from build123d import *

# Parameters (mm, degrees)
SKETCH1_R                = 19.05
BOSS_EXTRUDE1_DEPTH      = 203.2
SKETCH2_R                = 33.02
BOSS_EXTRUDE2_DEPTH      = 1
BOSS_EXTRUDE3_START      = 1.016
SKETCH3_R                = 33.02
BOSS_EXTRUDE3_DEPTH      = 1.016
SHELL2_START             = -0.016
SHELL2_OUTLINE_R         = 18.05
SHELL2_DEPTH             = 204.216
BOSS_EXTRUDE4_REACH      = 235.917
BOSS_EXTRUDE4_END_RADIUS = 19.05
SKETCH4_R                = 6.35
CUT_EXTRUDE1_REACH       = 235.917
CUT_EXTRUDE1_END_RADIUS  = 18.05
SKETCH5_R                = 5.08
BOSS_EXTRUDE5_REACH      = 258.931
BOSS_EXTRUDE5_END_RADIUS = 19.05
SKETCH6_R                = 6.35
CUT_EXTRUDE3_REACH       = 223.383
SKETCH8_R                = 4
BOSS_EXTRUDE6_START      = 50.8
SKETCH9_R                = 6.35
BOSS_EXTRUDE6_DEPTH      = 255.016
CUT_EXTRUDE2_REACH       = 258.931
CUT_EXTRUDE2_END_RADIUS  = 18.05
SKETCH7_R                = 5.08
SKETCH11_R               = 44.45
BOSS_EXTRUDE7_DEPTH      = 1
CUT_EXTRUDE5_REACH       = 272.789
SKETCH13_R               = 2.032
CUT_EXTRUDE6_REACH       = 272.789
SKETCH15_R               = 5.08
FILLET1_R                = 0.254


# Read off the part's stored shape, not the designer's step: Shell2
with BuildPart() as part:
    # Sketch1 → Boss-Extrude1 (new body)
    with BuildSketch(Plane(origin=(0, 0, 0), x_dir=(1, 0, 0), z_dir=(0, 1, 0))):
        with Locations(Location((0, 0, 0), (0, 0, 270))):
            Circle(SKETCH1_R)
    extrude(amount=BOSS_EXTRUDE1_DEPTH)

    # Sketch2 → Boss-Extrude2 (add)
    with BuildSketch(Plane(origin=(0, 203.2, 0), x_dir=(1, 0, 0), z_dir=(0, 1, 0))):
        with Locations(Location((0, 0, 0), (0, 0, 270))):
            Circle(SKETCH2_R)
    extrude(amount=BOSS_EXTRUDE2_DEPTH)

    # Sketch3 → Boss-Extrude3 (add)
    with BuildSketch(Plane.XZ.offset(BOSS_EXTRUDE3_START)):
        with Locations(Location((0, 0, 0), (0, 0, 90))):
            Circle(SKETCH3_R)
    extrude(amount=-BOSS_EXTRUDE3_DEPTH)

    # Shell2 outline → Shell2 (cut)
    with BuildSketch(Plane(origin=(0, 0, 0), x_dir=(1, 0, 0), z_dir=(0, 1, 0)).offset(SHELL2_START)):
        Circle(SHELL2_OUTLINE_R)
    extrude(amount=SHELL2_DEPTH, mode=Mode.SUBTRACT)

    # Boss-Extrude4: up to this cylinder (the profile starts outside it)
    boss_extrude4_end = Plane(origin=(0, 189.341, 0), z_dir=(0, -1, 0)) * Cylinder(BOSS_EXTRUDE4_END_RADIUS, 510.934, mode=Mode.PRIVATE)
    # Sketch4 → Boss-Extrude4 (add, up to the surface)
    with BuildSketch(Plane(origin=(-76.2, 0, 0), x_dir=(0, 0, -1), z_dir=(1, 0, 0)), mode=Mode.PRIVATE) as boss_extrude4_sk1:
        with Locations(Location((0, 189.341, 0), (0, 0, 180))):
            Circle(SKETCH4_R)
    boss_extrude4_tool1 = extrude(boss_extrude4_sk1.sketch, amount=BOSS_EXTRUDE4_REACH, mode=Mode.PRIVATE) - boss_extrude4_end
    add(boss_extrude4_tool1.solids().sort_by_distance((-76.2, 189.341, 0))[0])

    # Cut-Extrude1: up to this cylinder (the profile starts outside it)
    cut_extrude1_end = Plane(origin=(0, 189.341, 0), z_dir=(0, -1, 0)) * Cylinder(CUT_EXTRUDE1_END_RADIUS, 508.934, mode=Mode.PRIVATE)
    # Sketch5 → Cut-Extrude1 (cut, up to the surface)
    with BuildSketch(Plane.ZY.offset(76.2), mode=Mode.PRIVATE) as cut_extrude1_sk1:
        with Locations((0, 189.341)):
            Circle(SKETCH5_R)
    cut_extrude1_tool1 = extrude(cut_extrude1_sk1.sketch, amount=-CUT_EXTRUDE1_REACH, mode=Mode.PRIVATE) - cut_extrude1_end
    add(cut_extrude1_tool1.solids().sort_by_distance((-76.2, 189.341, 0))[0], mode=Mode.SUBTRACT)

    # Boss-Extrude5: up to this cylinder (the profile starts outside it)
    boss_extrude5_end = Plane(origin=(0, 10.16, 0), z_dir=(0, -1, 0)) * Cylinder(BOSS_EXTRUDE5_END_RADIUS, 556.962, mode=Mode.PRIVATE)
    # Sketch6 → Boss-Extrude5 (add, up to the surface)
    with BuildSketch(Plane(origin=(76.2, 0, 0), x_dir=(0, 0, -1), z_dir=(1, 0, 0)), mode=Mode.PRIVATE) as boss_extrude5_sk1:
        with Locations((0, 10.16)):
            Circle(SKETCH6_R)
    boss_extrude5_tool1 = extrude(boss_extrude5_sk1.sketch, amount=-BOSS_EXTRUDE5_REACH, mode=Mode.PRIVATE) - boss_extrude5_end
    add(boss_extrude5_tool1.solids().sort_by_distance((76.2, 10.16, 0))[0])

    # Sketch8 → Cut-Extrude3 (cut, up to next)
    with BuildSketch(Plane.XZ.offset(1.016), mode=Mode.PRIVATE) as cut_extrude3_sk1:
        with Locations(Location((0, 0, 0), (0, 0, 270))):
            Circle(SKETCH8_R)
    cut_extrude3_tool1 = extrude(cut_extrude3_sk1.sketch, amount=-CUT_EXTRUDE3_REACH, mode=Mode.PRIVATE) & part.part
    add(cut_extrude3_tool1.solids().sort_by_distance((0, -1.016, 0))[0], mode=Mode.SUBTRACT)

    # Sketch9 → Boss-Extrude6 (add)
    with BuildSketch(Plane.XZ.offset(1.016).offset(BOSS_EXTRUDE6_START)):
        with Locations(Location((0, 0, 0), (0, 0, 270))):
            Circle(SKETCH9_R)
    extrude(amount=-BOSS_EXTRUDE6_DEPTH)

    # Cut-Extrude2: up to this cylinder (the profile starts outside it)
    cut_extrude2_end = Plane(origin=(0, 10.16, 0), z_dir=(0, -1, 0)) * Cylinder(CUT_EXTRUDE2_END_RADIUS, 554.962, mode=Mode.PRIVATE)
    # Sketch7 → Cut-Extrude2 (cut, up to the surface)
    with BuildSketch(Plane(origin=(76.2, 0, 0), x_dir=(0, 0, -1), z_dir=(1, 0, 0)), mode=Mode.PRIVATE) as cut_extrude2_sk1:
        with Locations((0, 10.16)):
            Circle(SKETCH7_R)
    cut_extrude2_tool1 = extrude(cut_extrude2_sk1.sketch, amount=-CUT_EXTRUDE2_REACH, mode=Mode.PRIVATE) - cut_extrude2_end
    add(cut_extrude2_tool1.solids().sort_by_distance((76.2, 10.16, 0))[0], mode=Mode.SUBTRACT)

    # Sketch11 → Boss-Extrude7 (add)
    with BuildSketch(Plane(origin=(0, 204.2, 0), x_dir=(1, 0, 0), z_dir=(0, 1, 0))):
        with Locations(Location((0, 0, 0), (0, 0, 270))):
            Circle(SKETCH11_R)
    extrude(amount=-BOSS_EXTRUDE7_DEPTH)

    # Sketch13 → Cut-Extrude5 (cut, up to next)
    with BuildSketch(Plane(origin=(0, 204.2, 0), x_dir=(1, 0, 0), z_dir=(0, 1, 0)), mode=Mode.PRIVATE) as cut_extrude5_sk1:
        with Locations(Location((33.02, 0, 0), (0, 0, 270))):
            Circle(SKETCH13_R)
    cut_extrude5_tool1 = extrude(cut_extrude5_sk1.sketch, amount=-CUT_EXTRUDE5_REACH, mode=Mode.PRIVATE) & part.part
    # Sketch13 → Cut-Extrude5 (cut, up to next)
    with BuildSketch(Plane(origin=(0, 204.2, 0), x_dir=(1, 0, 0), z_dir=(0, 1, 0)), mode=Mode.PRIVATE) as cut_extrude5_sk2:
        with Locations(Location((0, -33.02, 0), (0, 0, 270))):
            Circle(SKETCH13_R)
    cut_extrude5_tool2 = extrude(cut_extrude5_sk2.sketch, amount=-CUT_EXTRUDE5_REACH, mode=Mode.PRIVATE) & part.part
    # Sketch13 → Cut-Extrude5 (cut, up to next)
    with BuildSketch(Plane(origin=(0, 204.2, 0), x_dir=(1, 0, 0), z_dir=(0, 1, 0)), mode=Mode.PRIVATE) as cut_extrude5_sk3:
        with Locations(Location((-33.02, 0, 0), (0, 0, 270))):
            Circle(SKETCH13_R)
    cut_extrude5_tool3 = extrude(cut_extrude5_sk3.sketch, amount=-CUT_EXTRUDE5_REACH, mode=Mode.PRIVATE) & part.part
    # Sketch13 → Cut-Extrude5 (cut, up to next)
    with BuildSketch(Plane(origin=(0, 204.2, 0), x_dir=(1, 0, 0), z_dir=(0, 1, 0)), mode=Mode.PRIVATE) as cut_extrude5_sk4:
        with Locations(Location((0, 33.02, 0), (0, 0, 270))):
            Circle(SKETCH13_R)
    cut_extrude5_tool4 = extrude(cut_extrude5_sk4.sketch, amount=-CUT_EXTRUDE5_REACH, mode=Mode.PRIVATE) & part.part
    add(cut_extrude5_tool1.solids().sort_by_distance((33.02, 204.2, 0))[0], mode=Mode.SUBTRACT)
    add(cut_extrude5_tool2.solids().sort_by_distance((0, 204.2, 33.02))[0], mode=Mode.SUBTRACT)
    add(cut_extrude5_tool3.solids().sort_by_distance((-33.02, 204.2, 0))[0], mode=Mode.SUBTRACT)
    add(cut_extrude5_tool4.solids().sort_by_distance((0, 204.2, -33.02))[0], mode=Mode.SUBTRACT)

    # Sketch15 → Cut-Extrude6 (cut, up to next)
    with BuildSketch(Plane.XZ.offset(51.816), mode=Mode.PRIVATE) as cut_extrude6_sk1:
        with Locations(Location((0, 0, 0), (0, 0, 270))):
            Circle(SKETCH15_R)
    cut_extrude6_tool1 = extrude(cut_extrude6_sk1.sketch, amount=-CUT_EXTRUDE6_REACH, mode=Mode.PRIVATE) & part.part
    add(cut_extrude6_tool1.solids().sort_by_distance((0, -51.816, 0))[0], mode=Mode.SUBTRACT)

    # Fillet1
    fillet1_edges = [part.edges().sort_by_distance(p)[0] for p in [
        (0, 204.2, 5.08),
    ]]
    fillet(fillet1_edges, radius=FILLET1_R)


solid = part.part
Check sheet for the modelled part. Datum: model origin and axes. Units: mm. A direction names the side the tool comes from. Round coordinates to 2 decimals unless told otherwise and drop trailing zeros. Order: outer loops, then holes, each group sorted by start corner. A loop starts at its lowest first (then second) coordinate and runs counter-clockwise, first axis right, second up.
(1) Cross-section at B-B, the plane z = 22. Enter the section's corners in (x, y), and give its area (3 significant figures).
(2) Cross-section at A-A, the plane y = 10.16. Enter the section's corners in (x, z), and give its area (3 significant figures).
(3) Access from +Z, -Z, +X, -X, +Y, -Y to the whole of each face (thin tool, end or side, straight path). Record for faces 1 (the cylindrical face through (47.49, 3.96, 1.38)), 2 (the cylindrical face through (-3.86, -26.77, 5.04)), 3 (the flat face through (0, -0.016, 8)).
(4) Cross-section at D-D, the plane x = -40.5. Enter the section's corners in (y, z).
(5) Cross-section at C-C, the plane y = 94.5. Enter the section's corners in (x, z).
(6) Scan lines: probe 1 along Y at (x, z) = (61, 0); probe 2 along Y at (x, z) = (-0.5, -12); probe 3 along X at (y, z) = (203.7, 0). Record each from-to range of solid material in increasing order.
(7) Go/stop test with flat-tipped pins: P1, Ø3.5, axis at x = 0, z = -33.02, coming from the +Y side; P2, Ø4.5, axis at x = 33.02, z = 0, coming from the +Y side; P3, Ø4, axis at x = -21.5, z = -14.5, coming from the -Y side; P4, Ø9, axis at y = 189.341, z = 0, coming from the -X side. Record where each tip stops, or that it passes through.
(8) Draft check along X on faces 4 (the flat face through (0, 203.2, 8)), 5 (the cylindrical face through (-47.172, 194.378, -0.661)), 6 (the flat face through (76.2, 15, -2)). Enter one of: pulls with the +X half, pulls with the -X half, needs draft (parallel to the pull), parting line crosses it, or undercut.
Check sheet entries:
1. outline: (-38.62, 203.2) - (38.62, 203.2) - (38.62, 204.2) - (-38.62, 204.2) - close; (-24.62, -1.02) - (24.62, -1.02) - (24.62, 0) - (-24.62, 0) - close
1. area: 127 mm2
2. outline: circle Ø12.7 at (0, 0); (17.32, -5.08) arc R18.05 cw (long way) to (17.32, 5.08) - (76.2, 5.08) - (76.2, 6.35) - (17.96, 6.35) arc R19.05 ccw (long way) to (17.96, -6.35) - (76.2, -6.35) - (76.2, -5.08) - close; hole circle Ø10.16 at (0, 0)
2. area: 299 mm2
3. face 1: +X
3. face 2: -Y
3. face 3: none
4. outline: circle Ø12.7 at (189.34, 0); (203.2, -18.32) - (204.2, -18.32) - (204.2, 18.32) - (203.2, 18.32) - close; hole circle Ø10.16 at (189.34, 0)
5. outline: circle Ø38.1 at (0, 0); circle Ø12.7 at (0, 0); hole circle Ø36.1 at (0, 0); hole circle Ø10.16 at (0, 0)
6. probe 1: y = 3.81 to 5.08, 15.24 to 16.51
6. probe 2: y = -1.02 to -0.02, 203.2 to 204.2
6. probe 3: x = -44.45 to -35.05, -30.99 to -5.08, 5.08 to 30.99, 35.05 to 44.45
7. P1: stops at y = 0
7. P2: stops at y = 204.2
7. P3: stops at y = -1.02
7. P4: stops at x = -6.35
8. face 4: undercut
8. face 5: needs draft
8. face 6: pulls with the +X half
